from build123d import *

# Parameters (mm, degrees)
BOSS_EXTRUDE1_DEPTH = 3.175
SKETCH5_R           = 0.79375
CUT_EXTRUDE10_DEPTH = 19.05


with BuildPart() as part:
    # Sketch2 → Boss-Extrude1 (new body)
    with BuildSketch(Plane.XY):
        with BuildLine():
            Line((76.2, 0), (76.2, -76.2))
            Line((76.2, -76.2), (37.846, -76.2))
            ThreePointArc((37.846, -76.2), (11.084836759, -65.115163241), (0, -38.354))
            Line((0, -38.354), (0, -37.846))
            ThreePointArc((0, -37.846), (11.084836759, -11.084836759), (37.846, 0))
            Line((37.846, 0), (76.2, 0))
        make_face()
    extrude(amount=BOSS_EXTRUDE1_DEPTH)

    # Sketch5 → Cut-Extrude10 (cut)
    with BuildSketch(Plane.XY):
        with Locations((38.1, -38.1)):
            Circle(SKETCH5_R)
        with Locations((66.675, -38.1)):
            Circle(SKETCH5_R)
        with Locations((62.846675913, -52.3875)):
            Circle(SKETCH5_R)
        with Locations((52.3875, -62.846675913)):
            Circle(SKETCH5_R)
        with Locations((38.1, -66.675)):
            Circle(SKETCH5_R)
        with Locations((23.8125, -62.846675913)):
            Circle(SKETCH5_R)
        with Locations((13.353324087, -52.3875)):
            Circle(SKETCH5_R)
        with Locations((9.525, -38.1)):
            Circle(SKETCH5_R)
        with Locations((13.353324087, -23.8125)):
            Circle(SKETCH5_R)
        with Locations((23.8125, -13.353324087)):
            Circle(SKETCH5_R)
        with Locations((38.1, -9.525)):
            Circle(SKETCH5_R)
        with Locations((52.3875, -13.353324087)):
            Circle(SKETCH5_R)
        with Locations((62.846675913, -23.8125)):
            Circle(SKETCH5_R)
    extrude(amount=CUT_EXTRUDE10_DEPTH, mode=Mode.SUBTRACT)


solid = part.part
Input: part model. Units: mm. Frame: model coordinates. Round coordinates to 2 decimals unless told otherwise and drop trailing zeros. Loops run counter-clockwise (first coordinate to the right, second up) from the corner with the lowest first, then second, coordinate; pieces in that order, holes last. Notation, with made-up numbers: M 23.25,-12 L 38.25,-12 A14 ccw 38.25,11 Z; hole C 53,3.25 d8. An arc over 180 degrees is marked long. Answer as CSV lines item,"result". Start each with the question number.
(1) Section A-A, the plane z = 2.2. State how many separate pieces and enclosed holes the cut face has, plus the area to 3 significant figures.
(2) Line query: line 1 (X direction, y = -38, z = 0.35); line 2 (Y direction, x = 63, z = 2.6); line 3 (Y direction, x = 37.5, z = 2.2). Output: solid intervals per line, ascending. Write a range as [from, to].
(3) Draft query along Z for faces 1 (the flat face through (76.2, -38, 2)), 2 (the flat face through (47, -38, 3.175)), 3 (the flat face through (47, -38, 0)). Return one class per face: released by +Z, released by -Z, zero draft, split by the parting line, or undercut.
(4) Section B-B, the plane y = -19. Output: boundary loops of the cut face in (x, z) (3 decimals), plus the area to 3 significant figures.
Values found:
1,separate pieces,"1"
1,enclosed holes,"13"
1,area,"5,170 mm²"
2,line 1,"x = [0, 8.74], [10.31, 37.31], [38.89, 65.89], [67.46, 76.2]"
2,line 2,"y = [-76.2, -53.17], [-51.61, -24.59], [-23.03, 0]"
2,line 3,"y = [-76.2, -67.19], [-66.16, -38.62], [-37.58, -10.04], [-9.01, 0]"
3,face 1,"zero draft"
3,face 2,"released by +Z"
3,face 3,"released by -Z"
4,outline,"M 5.026,0 L 76.2,0 L 76.2,3.175 L 5.026,3.175 Z"
4,area,"226 mm²"
